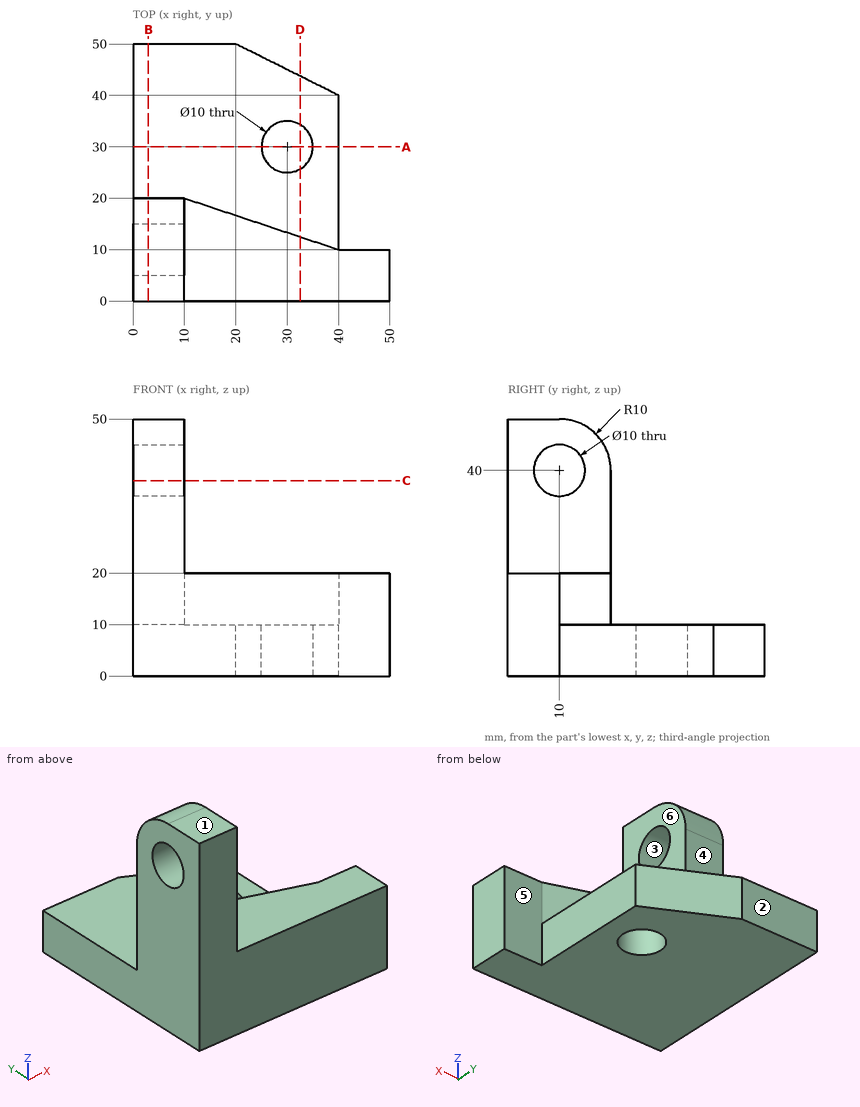
Geometry check sheet. Reference: drawing and pictorial views, mm from the part's lowest x, y, z. A direction names the side the tool comes from. Coordinates: 2 decimals unless noted, no trailing zeros. Order: outer loops, then holes, each group sorted by start corner. A loop starts at its lowest first (then second) coordinate and runs counter-clockwise, first axis right, second up. Notation, with made-up numbers: M 84.25,75.5 L 113.25,75.5 A18 ccw 113.25,87.5 Z; hole C 36.25,-13 d4. An arc over 180 degrees is marked long. Return JSON: item names as keys, results as strings.
1) Thickness scan on L1, parallel to Y at x = 3.25, z = 40; L2, parallel to Y at x = 30, z = 4.25; L3, parallel to Z at x = 14, y = 14. Record the ranges inside material, lowest first. Write a range as [from, to].
Answer list:
{"L1": "[0, 5], [15, 20]", "L2": "[0, 25], [35, 45]", "L3": "[0, 20]"}
2) Cross-section at B-B, the plane x = 3. Record the boundary of the cut face in (y, z).
Answer list:
{"outline": "M 0,0 L 50,0 L 50,10 L 20,10 L 20,40 A10 ccw 10,50 L 0,50 Z; hole C 10,40 d10"}
3) Access from +Z, -Z, +X, -X, +Y, -Y to the whole of each face (thin tool, end or side, straight path). Record for the marked faces 4, 5 and 6.
Answer list:
{"face 4": "+Z, +X, -X, +Y", "face 5": "+Z, -Z, +X, +Y", "face 6": "+Z, +X, +Y, -Y"}
4) Cross-section at C-C, the plane z = 38. Record the boundary of the cut face in (x, y), and give its area (3 significant figures).
Answer list:
{"outline": "M 0,0 L 10,0 L 10,5.42 L 0,5.42 Z; M 0,14.58 L 10,14.58 L 10,20 L 0,20 Z", "area": "108 mm2"}
5) Gauge pin test, flat ends, axial feed: pin 1 (3 mm diameter, centred on y = 13, z = 32, fed in from +X); pin 2 (6 mm diameter, centred on y = 45, z = 8, fed in from +X); pin 3 (1.5 mm diameter, centred on x = 20.5, y = 12.5, fed in from +Z). Record the tip position at first contact, or that the pin passes through.
Answer list:
{"pin 1": "x = 10", "pin 2": "x = 36", "pin 3": "z = 20"}
6) Release check for a two-part mould opening along Z. For the marked faces 1, 2 and 3 record: +Z half, -Z half, draft (parallel to the pull), parting line (faces both ways), or undercut.
Answer list:
{"face 1": "+Z half", "face 2": "draft", "face 3": "undercut"}
7) Cross-section at D-D, the plane x = 32.5. Record the boundary of the cut face in (y, z).
Answer list:
{"outline": "M 0,0 L 25.67,0 L 25.67,10 L 12.5,10 L 12.5,20 L 0,20 Z; M 34.33,0 L 43.75,0 L 43.75,10 L 34.33,10 Z"}
8) Cross-section at A-A, the plane y = 30. Record the boundary of the cut face in (x, z), and give its area (3 significant figures).
Answer list:
{"outline": "M 0,0 L 25,0 L 25,10 L 0,10 Z; M 35,0 L 40,0 L 40,10 L 35,10 Z", "area": "300 mm2"}
